Here's how the part is built. I have some questions about the finished solid (model axes, mm). A direction names the side the tool comes from. Round coordinates to 2 decimals unless told otherwise and drop trailing zeros. Write each loop counter-clockwise with the first axis right and the second up, starting at its lowest first coordinate (ties: lowest second). Pieces come first, ordered by that corner, then holes. Notation, with made-up numbers: M -14,58.5 L 10,58.5 A29 cw 10,91.5 Z; hole C 21,6 d10. An arc over 180 degrees is marked long. Use one line per item in the form item = value. Start each with the question number.
Q1. I want a section at A-A on z = 19.05. List the corners of the cut face in (x, y) for me.
Q2. For faces 4 (the face through (0.092, 29.565, 3.219)), 5 (the face through (-8, 19, 0)), 6 (the face through (-4, 29, 6.35)), which set-ups out of +Z, -Z, +X, -X, +Y, -Y let a thin tool reach every point of the face, with its end or its side?
Q3. I'm going to push flat-ended pins straight in: pin 1 Ø8 at (x, z) = (11.5, 33) entering from +Y; pin 2 Ø8.5 at (x, y) = (4.5, 25) entering from +Z; pin 3 Ø13.5 at (x, z) = (0, 19.05) entering from -Y; pin 4 Ø2 at (x, y) = (-8.5, 4.5) entering from +Z. Where does each tip first touch, or does it pass through?
Q4. We'd pull the mould along X, two halves only. Please class faces 1 (the face through (-16.637, 9, 8)), 2 (the face through (4.166, 19, 3)), 3 (the face through (16.637, 9, 8)): +X half, -X half, draft (parallel to the pull), parting line (faces both ways), or undercut.
Q5. I want a section at B-B on x = 0. List the corners of the cut face in (y, z) for me, and give its area (3 significant figures).
Q6. I want a section at D-D on x = 9. List the corners of the cut face in (y, z) for me.
Q7. I need wall thicknesses on line 1 along X through (y, z) = (2, 19); line 2 along Y through (x, z) = (10, 30); line 3 along Z through (x, y) = (0, 1). Which ranges of each line are inside material? Lowest first, please. Write a range as from..to.
```python
from build123d import *

# Parameters (mm, degrees)
BOSS_EXTRUDE1_DEPTH          = 33.274
CUT_EXTRUDE1_DEPTH           = 53.31120596
F_5_16_CLEARANCE_HOLE1_D     = 8.3312
F_5_16_CLEARANCE_HOLE1_DEPTH = 38.1
FILLET1_START                = -16.637
FILLET1_DEPTH                = 12.4714
FILLET1_START_2              = 4.1656
FILLET1_2_DEPTH              = 12.4714
FILLET1_START_3              = 6.35
FILLET1_3_DEPTH              = 7.9248
FILLET1_START_4              = -4.1656
FILLET1_4_DEPTH              = 8.3312


with BuildPart() as part:
    # Sketch1 → Boss-Extrude1 (new body)
    with BuildSketch(Plane(origin=(-16.637, 0, 0), x_dir=(0, -1, 0), z_dir=(-1, 0, 0))):
        with BuildLine():
            Line((-6.35, 31.75), (-6.35, 6.35))
            Line((-6.35, 6.35), (-31.75, 6.35))
            ThreePointArc((-31.75, 6.35), (-36.240128061, 4.490128061), (-38.1, 0))
            Line((-38.1, 0), (0, 0))
            Line((0, 0), (0, 38.1))
            ThreePointArc((0, 38.1), (-4.490128061, 36.240128061), (-6.35, 31.75))
        make_face()
    extrude(amount=-BOSS_EXTRUDE1_DEPTH)

    # Sketch2 → Cut-Extrude1 (cut, through all)
    with BuildSketch(Plane.XY.offset(6.35)):
        with BuildLine():
            Line((4.1656, 12.7), (4.1656, 25.4))
            ThreePointArc((4.1656, 25.4), (0, 29.5656), (-4.1656, 25.4))
            Line((-4.1656, 25.4), (-4.1656, 12.7))
            ThreePointArc((-4.1656, 12.7), (0, 8.5344), (4.1656, 12.7))
        make_face()
    extrude(amount=-CUT_EXTRUDE1_DEPTH, mode=Mode.SUBTRACT)

    # 5/16 Clearance Hole1
    with Locations(Plane(origin=(0, 0, 0), x_dir=(-1, 0, 0), z_dir=(0, -1, 0))):
        with Locations((0, -19.05)):
            Hole(F_5_16_CLEARANCE_HOLE1_D / 2, depth=F_5_16_CLEARANCE_HOLE1_DEPTH)

    # Fillet1: read off the stored shape, not the designer's step
    # Fillet1 outline → Fillet1 (add)
    with BuildSketch(Plane.YZ.offset(FILLET1_START)):
        with BuildLine():
            ThreePointArc((14.2748, 6.35), (8.67112018, 8.67112018), (6.35, 14.2748))
            Line((6.35, 14.2748), (6.35, 6.35))
            Line((6.35, 6.35), (14.2748, 6.35))
        make_face()
    extrude(amount=FILLET1_DEPTH)

    # Fillet1 2 outline → Fillet1 2 (add)
    with BuildSketch(Plane.YZ.offset(FILLET1_START_2)):
        with BuildLine():
            ThreePointArc((14.2748, 6.35), (8.67112018, 8.67112018), (6.35, 14.2748))
            Line((6.35, 14.2748), (6.35, 6.35))
            Line((6.35, 6.35), (14.2748, 6.35))
        make_face()
    extrude(amount=FILLET1_2_DEPTH)

    # Fillet1 3 outline → Fillet1 3 (add)
    with BuildSketch(Plane.XY.offset(FILLET1_START_3)):
        with BuildLine():
            ThreePointArc((4.1656, 12.7), (0, 8.5344), (-4.1656, 12.7))
            Line((-4.1656, 12.7), (-4.1656, 6.35))
            Line((-4.1656, 6.35), (4.1656, 6.35))
            Line((4.1656, 6.35), (4.1656, 12.7))
        make_face()
    extrude(amount=FILLET1_3_DEPTH)

    # Fillet1 4 outline → Fillet1 4 (cut)
    with BuildSketch(Plane.YZ.offset(FILLET1_START_4)):
        with BuildLine():
            Line((14, 14.2748), (6.35, 14.2748))
            ThreePointArc((6.35, 14.2748), (8.574791663, 8.769133827), (14, 6.354765909))
            Line((14, 6.354765909), (14, 14.2748))
        make_face()
    extrude(amount=FILLET1_4_DEPTH, mode=Mode.SUBTRACT)


solid = part.part
```
Reported:
q1.outline = M -16.64,0 L -4.17,0 L -4.17,6.35 L -16.64,6.35 Z; M 4.17,0 L 16.64,0 L 16.64,6.35 L 4.17,6.35 Z
q2.face_4 = +Z, -Z
q2.face_5 = -Z, +X, -X, +Y, -Y
q2.face_6 = +Z, +X, -X, +Y
q3.pin_1 = 6.35
q3.pin_2 = 6.35
q3.pin_3 = 0
q3.pin_4 = 37.05
q4.face_1 = -X half
q4.face_2 = undercut
q4.face_3 = +X half
q5.outline = M 0,0 L 8.53,0 L 8.53,8.81 A7.92 cw 6.35,14.27 L 6.35,14.88 L 0,14.88 Z; M 0,23.22 L 6.35,23.22 L 6.35,31.75 A6.35 ccw 0,38.1 Z; M 29.57,0 L 38.1,0 A6.35 ccw 31.75,6.35 L 29.57,6.35 Z
q5.area = 249 mm^2
q6.outline = M 0,0 L 38.1,0 A6.35 ccw 31.75,6.35 L 14.27,6.35 A7.92 cw 6.35,14.27 L 6.35,31.75 A6.35 ccw 0,38.1 Z
q7.line_1 = -16.64..-4.17, 4.17..16.64
q7.line_2 = 0..6.35
q7.line_3 = 0..14.88, 23.22..38.02
